Geometry: final body of the model. Coordinates: model frame, mm. A direction names the side the tool comes from. Coordinates: 2 decimals unless noted, no trailing zeros. Write each loop counter-clockwise with the first axis right and the second up, starting at its lowest first coordinate (ties: lowest second). Pieces come first, ordered by that corner, then holes. Notation, with made-up numbers: (-18, 82) - (0, 82) arc R26 ccw to (0, 119) - close; hole circle Ø4 at (-19, -23). An arc over 180 degrees is marked (long way). Put each result on its own line as item: value.
```python
from build123d import *

# Parameters (mm, degrees)
PAD_DEPTH       = 480
POCKET_DEPTH    = 59.501
POCKET001_DEPTH = 59.501


with BuildPart() as part:
    # Sketch → Pad (new body)
    with BuildSketch(Plane.XY):
        Polygon((-29.75, 25), (-29.75, 0), (29.75, 0), (29.75, 25), (28.583333, 25), (28.583333, 1.166667), (0.583333, 1.166667), (0.583333, 25), (-0.583333, 25), (-0.583333, 1.166667), (-28.583333, 1.166667), (-28.583333, 25), align=None)
    extrude(amount=PAD_DEPTH)

    # Sketch001 (on Face3 of Pad) → Pocket (cut, through all)
    with BuildSketch(Plane.YZ.offset(29.75)):
        Polygon((0, 0), (25, 25), (25, 0), align=None)
    extrude(amount=-POCKET_DEPTH, mode=Mode.SUBTRACT)

    # Sketch002 (on Face6 of Pocket) → Pocket001 (cut, through all)
    with BuildSketch(Plane.YZ.offset(29.75)):
        Polygon((0, 480), (25, 455), (25, 480), align=None)
    extrude(amount=-POCKET001_DEPTH, mode=Mode.SUBTRACT)


solid = part.part
```
1. Mould query, pull axis X, two halves, no side actions, for faces 3 (the flat face through (-0.583, 13, 237)), 4 (the flat face through (0, 9, 9)), 5 (the flat face through (29.75, 12, 237)), 6 (the flat face through (15, 1.167, 237)). Classes: +X half, -X half, draft (parallel to the pull), parting line (faces both ways), or undercut.
Answer below:
face 3: undercut
face 4: draft
face 5: +X half
face 6: undercut
2. Section query C-C (x = -24.5). Return loops of the section in (y, z), then the cut area to 3 significant figures.
Answer below:
outline: (0, 0) - (1.17, 1.17) - (1.17, 478.83) - (0, 480) - close
area: 559 mm²
3. Set-up query: faces 1 (the flat face through (0.583, 13, 237)), 2 (the flat face through (0, 9, 471)). Return all of +Z, -Z, +X, -X, +Y, -Y with unobstructed straight access to the full face (end or side cutting, diameter ignored); none if empty.
Answer below:
face 1: +Z, -Z, +Y
face 2: +Z, +X, -X, +Y
4. Pin query (flat end, axial travel): pin 1 Ø14 at (x, z) = (16.5, 314) entering from +Y; pin 2 Ø5 at (x, y) = (-20, 6) entering from +Z. Return the tip coordinate at first contact, or that it passes through.
Answer below:
pin 1: stops at y = 1.17
pin 2: passes through
5. Section query B-B (z = 440.5). Return loops of the section in (x, y).
Answer below:
outline: (-29.75, 0) - (29.75, 0) - (29.75, 25) - (28.58, 25) - (28.58, 1.17) - (0.58, 1.17) - (0.58, 25) - (-0.58, 25) - (-0.58, 1.17) - (-28.58, 1.17) - (-28.58, 25) - (-29.75, 25) - close
6. Section query A-A (y = 14.75). Return loops of the section in (x, z), then the cut area to 3 significant figures.
Answer below:
outline: (-29.75, 14.75) - (-28.58, 14.75) - (-28.58, 465.25) - (-29.75, 465.25) - close; (-0.58, 14.75) - (0.58, 14.75) - (0.58, 465.25) - (-0.58, 465.25) - close; (28.58, 14.75) - (29.75, 14.75) - (29.75, 465.25) - (28.58, 465.25) - close
area: 1,580 mm²
7. Ray query, probe 1 along X at (y, z) = (9.25, 183); probe 2 along Y at (x, z) = (14, 234.5); probe 3 along Z at (x, y) = (-20.5, 1). Return the intervals inside material, ascending. Write a range as from..to.
Answer below:
probe 1: x = -29.75..-28.58, -0.58..0.58, 28.58..29.75
probe 2: y = 0..1.17
probe 3: z = 1..479
